Read the model definition and answer for the solid it produces. Units are mm, in the model's axes. A direction names the side the tool comes from. Round coordinates to 2 decimals unless told otherwise and drop trailing zeros. Return JSON: item names as keys, results as strings.
from build123d import *

# Parameters (mm, degrees)
BOSS_EXTRUDE1_DEPTH      = 11.1125
BOSS_EXTRUDE1_DEPTH_BACK = 11.1125
SKETCH5_W                = 109.877468776
SKETCH5_H                = 283.051122129
CUT_EXTRUDE2_DEPTH       = 1193.492852366
SKETCH6_W                = 149.121482991
SKETCH6_H                = 108.921761737
CUT_EXTRUDE3_DEPTH       = 1175.662940665
SKETCH7_R                = 4.7625
CUT_EXTRUDE4_DEPTH       = 635
CUT_EXTRUDE8_DEPTH       = 1195.766301895
CUT_EXTRUDE8_DEPTH_BACK  = 1195.766301895
SKETCH8_W                = 149.774750394
SKETCH8_H                = 148.832770831
SKETCH8_H_2              = 142.875
SKETCH8_H_3              = 176.125878949
SKETCH11_R               = 1.5875
CUT_EXTRUDE9_DEPTH       = 12.7
CUT_EXTRUDE10_START      = -12.7
SKETCH12_R               = 1.5875
CUT_EXTRUDE10_DEPTH      = 12.7


with BuildPart() as part:
    # Sketch1 → Boss-Extrude1 (new, two sides: drawn at the far end of the back side and taken through both)
    with BuildSketch(Plane.XY.offset(-BOSS_EXTRUDE1_DEPTH_BACK)):
        Polygon((142.42123069, 465.168027231), (219.716026672, 465.168027231), (213.502471629, 1096.967634552), (181.068628681, 1174.337215652), (148.634785732, 1096.967634552), align=None)
    extrude(amount=BOSS_EXTRUDE1_DEPTH + BOSS_EXTRUDE1_DEPTH_BACK)

    # Sketch2 → Cut-Loft1 section 0
    with BuildSketch(Plane.XZ.offset(-465.168027231)):
        with BuildLine():
            Line((142.42123069, 0), (181.068628681, 11.1125))
            Line((181.068628681, 11.1125), (219.716026672, 0))
            Line((219.716026672, 0), (222.70513775, 0))
            Line((222.70513775, 0), (222.70513775, 15.258366339))
            Line((222.70513775, 15.258366339), (137.848628215, 15.258366339))
            Line((137.848628215, 15.258366339), (137.848628215, 0))
            Line((137.848628215, 0), (142.42123069, 0))
        make_face()
    # Sketch3 → Cut-Loft1 section 1
    with BuildSketch(Plane(origin=(0, 1096.967634552, 0), x_dir=(1, 0, 0), z_dir=(0, 1, 0))):
        with BuildLine():
            Line((213.502471629, 0), (181.068628681, -11.1125))
            Line((181.068628681, -11.1125), (148.634785732, 0))
            Line((148.634785732, 0), (137.848628215, 0))
            Line((137.848628215, 0), (137.848628215, -15.258366339))
            Line((137.848628215, -15.258366339), (222.70513775, -15.258366339))
            Line((222.70513775, -15.258366339), (222.70513775, 0))
            Line((222.70513775, 0), (213.502471629, 0))
        make_face()
    cut_loft1 = loft(mode=Mode.SUBTRACT)

    # Mirror1: Cut-Loft1 across plane
    add(cut_loft1.mirror(Plane.XY), mode=Mode.SUBTRACT)

    # Sketch5 → Cut-Extrude2 (cut, through all)
    with BuildSketch(Plane(origin=(-32.103098407, 13.457832356, 93.698704331), x_dir=(0.9470206004067627, 0.045661094409327196, 0.31791043842968925), z_dir=(-0.3211728232668741, 0.1346377834927197, 0.937401026696127))):
        with Locations((219.349244299, 1139.303724701)):
            Rectangle(SKETCH5_W, SKETCH5_H)
    cut_extrude2 = extrude(amount=CUT_EXTRUDE2_DEPTH, mode=Mode.SUBTRACT)

    # Sketch6 → Cut-Extrude3 (cut, through all)
    with BuildSketch(Plane(origin=(69.458274406, 29.117370568, 202.726547902), x_dir=(0.9470206004067623, -0.045661094409327495, -0.31791043842969063), z_dir=(0.3211728232668754, 0.13463778349272, 0.9374010266961263))):
        with Locations((131.752816965, 1118.922251835)):
            Rectangle(SKETCH6_W, SKETCH6_H)
    cut_extrude3 = extrude(amount=CUT_EXTRUDE3_DEPTH, mode=Mode.SUBTRACT)

    # Mirror2: Cut-Extrude2, Cut-Extrude3 across plane
    add(cut_extrude2.mirror(Plane.XY), mode=Mode.SUBTRACT)
    add(cut_extrude3.mirror(Plane.XY), mode=Mode.SUBTRACT)

    # Sketch7 → Cut-Extrude4 (cut)
    with BuildSketch(Plane.XZ.offset(-465.168027231)):
        with Locations(Location((181.068628681, 0, 0), (0, 0, 270))):
            Circle(SKETCH7_R)
    extrude(amount=-CUT_EXTRUDE4_DEPTH, mode=Mode.SUBTRACT)

    # Sketch8 → Cut-Extrude8 (cut, two sides: drawn at the far end of the back side and taken through both)
    with BuildSketch(Plane.XY.offset(-CUT_EXTRUDE8_DEPTH_BACK)):
        with Locations((180.5976389, 528.420830237)):
            Rectangle(SKETCH8_W, SKETCH8_H)
        with Locations((180.5976389, 817.149715652)):
            Rectangle(SKETCH8_W, SKETCH8_H_2)
        with Locations((180.5976389, 960.024715652)):
            Rectangle(SKETCH8_W, SKETCH8_H_2)
        with Locations((180.5976389, 1119.525155127)):
            Rectangle(SKETCH8_W, SKETCH8_H_3)
    extrude(amount=CUT_EXTRUDE8_DEPTH + CUT_EXTRUDE8_DEPTH_BACK, mode=Mode.SUBTRACT)

    # Sketch11 → Cut-Extrude9 (cut)
    with BuildSketch(Plane(origin=(0, 745.712215652, 0), x_dir=(1, 0, 0), z_dir=(0, 1, 0))):
        with Locations(Location((168.368628681, 0, 0), (0, 0, 270))):
            Circle(SKETCH11_R)
        with Locations(Location((193.768628681, 0, 0), (0, 0, 270))):
            Circle(SKETCH11_R)
    extrude(amount=-CUT_EXTRUDE9_DEPTH, mode=Mode.SUBTRACT)

    # Sketch12 → Cut-Extrude10 (cut)
    with BuildSketch(Plane.XZ.offset(-602.837215652).offset(CUT_EXTRUDE10_START)):
        with Locations(Location((168.368628681, 0, 0), (0, 0, 90))):
            Circle(SKETCH12_R)
        with Locations(Location((193.768628681, 0, 0), (0, 0, 90))):
            Circle(SKETCH12_R)
    extrude(amount=CUT_EXTRUDE10_DEPTH, mode=Mode.SUBTRACT)


solid = part.part
Item 1: Section A-A (y = 735.5) is taken. State how many separate pieces and enclosed holes the cut face has, then the cut area to 3 significant figures.
Worked answers:
{"separate pieces": "1", "enclosed holes": "3", "area": "713 mm2"}
Item 2: A tool of negligible diameter and unlimited length cuts with its end or side. For faces 4 (the flat face through (194, 733.012, 0)), 5 (the flat face through (181, 602.837, 5)), 6 (the cylindrical face through (195.32, 609.28, -0.34)), from which of +Z, -Z, +X, -X, +Y, -Y can it reach the whole face along a straight path? Write none if from no direction.
Worked answers:
{"face 4": "+Y", "face 5": "+Z, -Z, +X, -X, -Y", "face 6": "-Y"}
Item 3: Straight lines are drawn through the part: L1, parallel to Z at x = 196, y = 696.5; L2, parallel to Z at x = 157, y = 706. For each, find the intervals that lie inside material, in ascending order. Write a range as [from, to].
Worked answers:
{"L1": "z = [-6.55, 6.55]", "L2": "z = [-3.74, 3.74]"}
Item 4: For a pull along X with two mould halves and no side action, classify faces 1 (the flat face through (194, 615.537, 0)), 2 (the flat face through (181, 745.712, 5)), 3 (the cylindrical face through (195.343, 739.451, -0.207)) as released by +X, released by -X, zero draft, split by the parting line, or undercut.
Worked answers:
{"face 1": "undercut", "face 2": "zero draft", "face 3": "undercut"}
Item 5: Flat-ended cylindrical pins translate along their axes: pin 1 (8 mm diameter, centred on x = 170.5, y = 676.5, fed in from -Z); pin 2 (2.5 mm diameter, centred on x = 193.5, z = 0, fed in from -Y); pin 3 (3 mm diameter, centred on x = 187.5, y = 695, fed in from +Z); pin 4 (8.5 mm diameter, centred on x = 181.07, z = 0, fed in from -Y). Find the tip coordinate at first contact, or state that the pin passes through.
Worked answers:
{"pin 1": "stops at z = -9.12", "pin 2": "stops at y = 615.54", "pin 3": "stops at z = 9.61", "pin 4": "passes through"}
